For this review, take the finished solid that the model builds, in its own axes (mm). A direction names the side the tool comes from. Coordinates: 2 decimals unless noted, no trailing zeros. Write each loop counter-clockwise with the first axis right and the second up, starting at its lowest first coordinate (ties: lowest second). Pieces come first, ordered by that corner, then holes. Notation, with made-up numbers: M -30,-17 L 17,-17 A24 ccw 17,9 Z; hole C -8.75,12.5 d11. An arc over 180 degrees is marked long. One line per question, with ' | ' between items.
from build123d import *

# Parameters (mm, degrees)
SKETCH_1_R          = 25.4
SKETCH_1_R_2        = 10.5
EXTRUDE_1_DEPTH     = 2
CUT_EXTRUDE_1_DEPTH = 36.9766591
SKETCH_3_R          = 1.25
SKETCH_3_R_2        = 5
CUT_EXTRUDE_2_DEPTH = 36.269108296
FILLET_1_R          = 0.5


with BuildPart() as part:
    # 草图1 → 凸台-拉伸1 (new body)
    with BuildSketch(Plane(origin=(0, 0, 0), x_dir=(1, 0, 0), z_dir=(0, 1, 0))):
        with Locations(Location((0, 0, 0), (0, 0, 270))):
            Circle(SKETCH_1_R)
        with Locations(Location((0, 0, 0), (0, 0, 270))):
            Circle(SKETCH_1_R_2, mode=Mode.SUBTRACT)
    extrude(amount=EXTRUDE_1_DEPTH)

    # 草图2 → 切除-拉伸1 (cut, through all)
    with BuildSketch(Plane(origin=(0, 2, 0), x_dir=(1, 0, 0), z_dir=(0, 1, 0))):
        with BuildLine():
            Line((-7.1, 24.387496797), (-7.1, 14.762503203))
            ThreePointArc((-7.1, 14.762503203), (0, 13.75), (7.1, 14.762503203))
            Line((7.1, 14.762503203), (7.1, 24.387496797))
            ThreePointArc((7.1, 24.387496797), (0, 25.4), (-7.1, 24.387496797))
        make_face()
        with BuildLine():
            Line((17.57019176, 18.342528765), (9.234702798, 13.530031969))
            ThreePointArc((9.234702798, 13.530031969), (11.907849302, 6.875), (16.334702798, 1.232471235))
            Line((16.334702798, 1.232471235), (24.67019176, 6.044968031))
            ThreePointArc((24.67019176, 6.044968031), (21.997045256, 12.7), (17.57019176, 18.342528765))
        make_face()
        with BuildLine():
            Line((24.67019176, -6.044968031), (16.334702798, -1.232471235))
            ThreePointArc((16.334702798, -1.232471235), (11.907849302, -6.875), (9.234702798, -13.530031969))
            Line((9.234702798, -13.530031969), (17.57019176, -18.342528765))
            ThreePointArc((17.57019176, -18.342528765), (21.997045256, -12.7), (24.67019176, -6.044968031))
        make_face()
        with BuildLine():
            Line((7.1, -24.387496797), (7.1, -14.762503203))
            ThreePointArc((7.1, -14.762503203), (0, -13.75), (-7.1, -14.762503203))
            Line((-7.1, -14.762503203), (-7.1, -24.387496797))
            ThreePointArc((-7.1, -24.387496797), (0, -25.4), (7.1, -24.387496797))
        make_face()
        with BuildLine():
            Line((-17.57019176, -18.342528765), (-9.234702798, -13.530031969))
            ThreePointArc((-9.234702798, -13.530031969), (-11.907849302, -6.875), (-16.334702798, -1.232471235))
            Line((-16.334702798, -1.232471235), (-24.67019176, -6.044968031))
            ThreePointArc((-24.67019176, -6.044968031), (-21.997045256, -12.7), (-17.57019176, -18.342528765))
        make_face()
        with BuildLine():
            Line((-24.67019176, 6.044968031), (-16.334702798, 1.232471235))
            ThreePointArc((-16.334702798, 1.232471235), (-11.907849302, 6.875), (-9.234702798, 13.530031969))
            Line((-9.234702798, 13.530031969), (-17.57019176, 18.342528765))
            ThreePointArc((-17.57019176, 18.342528765), (-21.997045256, 12.7), (-24.67019176, 6.044968031))
        make_face()
    extrude(amount=-CUT_EXTRUDE_1_DEPTH, mode=Mode.SUBTRACT)

    # 草图3 → 切除-拉伸2 (cut, through all)
    with BuildSketch(Plane(origin=(0, 2, 0), x_dir=(1, 0, 0), z_dir=(0, 1, 0))):
        with Locations(Location((-10.25, 17.753520778, 0), (0, 0, 270))):
            Circle(SKETCH_3_R)
        with Locations(Location((10.25, 17.753520778, 0), (0, 0, 270))):
            Circle(SKETCH_3_R)
        with Locations(Location((20.5, 0, 0), (0, 0, 270))):
            Circle(SKETCH_3_R)
        with Locations(Location((10.25, -17.753520778, 0), (0, 0, 270))):
            Circle(SKETCH_3_R)
        with Locations(Location((-10.25, -17.753520778, 0), (0, 0, 270))):
            Circle(SKETCH_3_R)
        with Locations(Location((-20.5, 0, 0), (0, 0, 270))):
            Circle(SKETCH_3_R)
        with Locations((-29, 0)):
            Circle(SKETCH_3_R_2)
        with Locations((-14.5, 25.11473671)):
            Circle(SKETCH_3_R_2)
        with Locations((14.5, 25.11473671)):
            Circle(SKETCH_3_R_2)
        with Locations((29, 0)):
            Circle(SKETCH_3_R_2)
        with Locations((14.5, -25.11473671)):
            Circle(SKETCH_3_R_2)
        with Locations((-14.5, -25.11473671)):
            Circle(SKETCH_3_R_2)
    extrude(amount=-CUT_EXTRUDE_2_DEPTH, mode=Mode.SUBTRACT)

    # 圆角1
    fillet_1_edges = [part.edges().sort_by_distance(p)[0] for p in [
        (16.334702798, 1, -1.232471235),
        (9.234702798, 1, -13.530031969),
        (9.234702798, 1, 13.530031969),
        (16.334702798, 1, 1.232471235),
        (-7.1, 1, 14.762503203),
        (7.1, 1, 14.762503203),
        (-16.334702798, 1, 1.232471235),
        (-9.234702798, 1, 13.530031969),
        (-9.234702798, 1, -13.530031969),
        (-16.334702798, 1, -1.232471235),
        (7.1, 1, -14.762503203),
        (-7.1, 1, -14.762503203),
    ]]
    fillet(fillet_1_edges, radius=FILLET_1_R)


solid = part.part
1) To check wall thickness, follow line 1 along X through (y, z) = (0.75, 0); line 2 along Z through (x, y) = (16, 0.15); line 3 along X through (y, z) = (1.55, 4.5). State the ranges of each line that lie inside material, in increasing order. Write a range as [from, to].
Responses:
line 1: [-24, -21.75], [-19.25, -10.5], [10.5, 19.25], [21.75, 24] | line 2: [-19.73, -17.44], [-1.56, 1.56], [17.44, 19.73] | line 3: [-25, -21.99], [-13.46, -9.49], [9.49, 13.46], [21.99, 25]
2) Insertion check: pin 1 Ø0.6 at (y, z) = (1, 18) entering from -X; pin 2 Ø3 at (x, z) = (-18, -3) entering from +Y; pin 3 Ø0.6 at (y, z) = (1, 21) entering from +X; pin 4 Ø1 at (y, z) = (1.5, -17) entering from +X. Each pin has a flat end and moves straight along its axis. Give the tip position at first contact, or say it passes through.
Responses:
pin 1: x = -17.5 | pin 2: y = 2 | pin 3: x = 12.15 | pin 4: x = 16.11
3) We need section A-A on z = 0. State the section outline as (x, y) points, then the cut area to 3 significant figures.
Responses:
outline: M -24,0 L -21.75,0 L -21.75,2 L -24,2 Z; M -19.25,0 L -10.5,0 L -10.5,2 L -19.25,2 Z; M 10.5,0 L 19.25,0 L 19.25,2 L 10.5,2 Z; M 21.75,0 L 24,0 L 24,2 L 21.75,2 Z | area: 44.0 mm^2
4) We need section D-D on z = 7. State the section outline as (x, y) points, then the cut area to 3 significant figures.
Responses:
outline: M -11.84,0 L -7.83,0 L -7.83,2 L -11.84,2 Z; M 7.83,0 L 11.84,0 L 11.84,2 L 7.83,2 Z | area: 16.0 mm^2
5) Machinability: for faces 1 (the flat face through (-7.1, 1, 20)), 2 (the cylindrical face through (11.956, 1.014, 6.792)), 3 (the flat face through (-13.62, 1.01, 16.06)), which of the approach directions +Z, -Z, +X, -X, +Y, -Y give a long, thin tool a straight path to every point of the face, cutting with its end or side? Answer none if there is none.
Responses:
face 1: +Z, +Y, -Y | face 2: +Y, -Y | face 3: -X, +Y, -Y
6) We need section C-C on x = -6. State the section outline as (y, z) points, then the cut area to 3 significant figures.
Responses:
outline: M 0,-14.47 L 2,-14.47 L 2,-8.62 L 0,-8.62 Z; M 0,8.62 L 2,8.62 L 2,14.47 L 0,14.47 Z | area: 23.4 mm^2
7) We need section B-B on x = -12.5. State the section outline as (y, z) points.
Responses:
outline: M 0,-20.53 L 2,-20.53 L 2,-15.42 L 0,-15.42 Z; M 0,-5.9 L 2,-5.9 L 2,5.9 L 0,5.9 Z; M 0,15.42 L 2,15.42 L 2,20.53 L 0,20.53 Z
8) The part is to be moulded in two halves that separate along X. For faces 4 (the flat face through (-20.61, 1.01, 3.7)), 5 (the cylindrical face through (8.439, 0.986, 23.957)), 6 (the cylindrical face through (-16.5, 0.99, -19.31)), say which applies: +X half, -X half, draft (parallel to the pull), parting line (faces both ways), or undercut.
Responses:
face 4: undercut | face 5: +X half | face 6: -X half
